Geometry: see drawing. Coordinates: mm, zero at the bounding-box minimum. Round coordinates to 2 decimals unless told otherwise and drop trailing zeros. Loops run counter-clockwise (first coordinate to the right, second up) from the corner with the lowest first, then second, coordinate; pieces in that order, holes last. Notation, with made-up numbers: M 89.5,33 L 110.5,33 A13 ccw 110.5,55 Z; hole C -27.5,66 d3. An arc over 180 degrees is marked long. Answer as a JSON object with one key per item and string values.
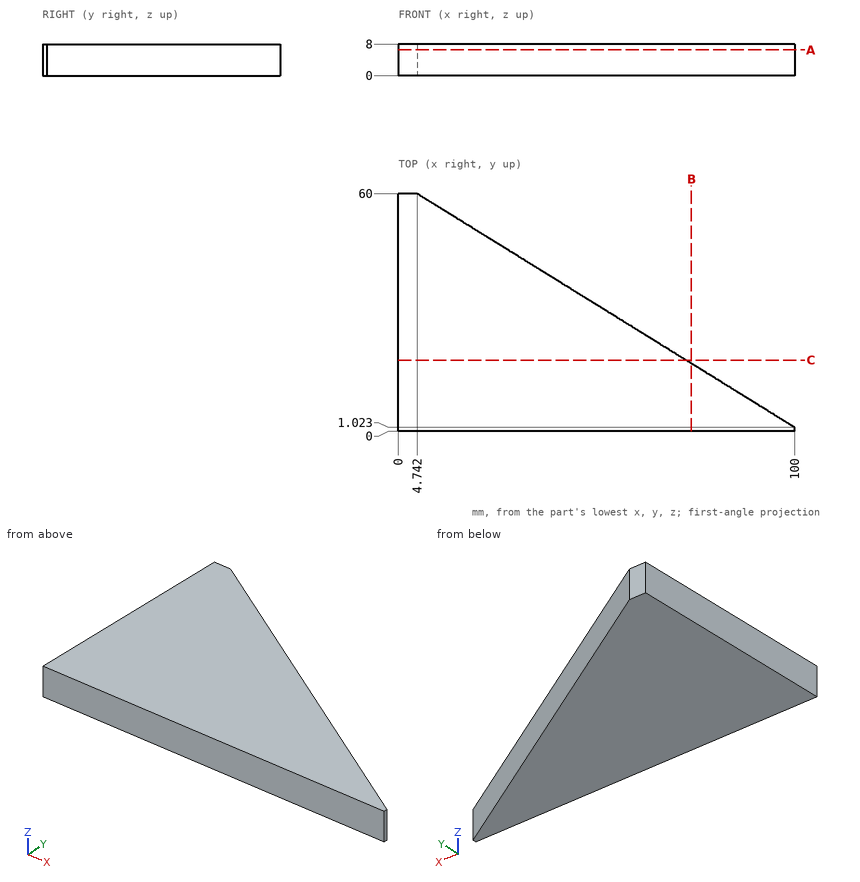
1) Section query B-B (x = 74). Return the cut outline in (y, z), and give its area (3 significant figures).
Results:
{"outline": "M 0,0 L 17.12,0 L 17.12,8 L 0,8 Z", "area": "137 mm2"}
2) Section query A-A (z = 6.5). Return the cut outline in (x, y).
Results:
{"outline": "M 0,0 L 100,0 L 100,1.02 L 4.74,60 L 0,60 Z"}
3) Pin query (flat end, axial travel): P1, Ø3, axis at y = 30.5, z = 3.5, coming from the +X side. Return the tip coordinate at first contact, or that it passes through.
Results:
{"P1": "x = 54.81"}
4) Ray query, line 1 (X direction, y = 15.5, z = 5); line 2 (X direction, y = 38, z = 5.5) (1 decimal); line 3 (Y direction, x = 46, z = 6.75). Return the intervals inside material, ascending.
Results:
{"line 1": "0 to 76.62", "line 2": "0 to 40.3", "line 3": "0 to 34.46"}
5) Section query C-C (y = 18). Return the cut outline in (x, z), and give its area (3 significant figures).
Results:
{"outline": "M 0,0 L 72.58,0 L 72.58,8 L 0,8 Z", "area": "581 mm2"}
